```python
from build123d import *

# Parameters (mm, degrees)
SKETCH1_R           = 7.5
BOSS_EXTRUDE1_DEPTH = 58
CUT_EXTRUDE1_REACH  = 42
CUT_EXTRUDE2_REACH  = 82
SKETCH3_R           = 7
CHAMFER1_SIZE       = 15
CUT_EXTRUDE3_DEPTH  = 6
SKETCH4_3_R         = 7.5
CUT_EXTRUDE4_DEPTH  = 12


with BuildPart() as part:
    # Sketch1 → Boss-Extrude1 (new body)
    with BuildSketch(Plane.XY):
        with BuildLine():
            Line((-34, -19), (31, -19))
            Line((31, -19), (46, -10.339745962))
            Line((46, -10.339745962), (46, 12.339745962))
            Line((46, 12.339745962), (31, 21))
            Line((31, 21), (2.66060556, 21))
            ThreePointArc((2.66060556, 21), (-17.33939444, 16.82575695), (-34, 5))
            Line((-34, 5), (-34, -19))
        make_face()
        Circle(SKETCH1_R, mode=Mode.SUBTRACT)
    extrude(amount=BOSS_EXTRUDE1_DEPTH)

    # Sketch2 → Cut-Extrude1 (cut, up to next)
    with BuildSketch(Plane.XZ.offset(19), mode=Mode.PRIVATE) as cut_extrude1_sk1:
        Polygon((-34, 50), (-18, 50), (-18, 44), (20, 44), (20, 14), (-18, 14), (-18, 8), (-34, 8), align=None)
    cut_extrude1_tool1 = extrude(cut_extrude1_sk1.sketch, amount=-CUT_EXTRUDE1_REACH, mode=Mode.PRIVATE) & part.part
    add(cut_extrude1_tool1.solids().sort_by_distance((-9.013245, -19, 29))[0], mode=Mode.SUBTRACT)

    # Sketch3 → Cut-Extrude2 (cut, up to next)
    with BuildSketch(Plane(origin=(46, 0, 0), x_dir=(0, 0, -1), z_dir=(1, 0, 0)), mode=Mode.PRIVATE) as cut_extrude2_sk1:
        with Locations((-29, 1)):
            Circle(SKETCH3_R)
    cut_extrude2_tool1 = extrude(cut_extrude2_sk1.sketch, amount=-CUT_EXTRUDE2_REACH, mode=Mode.PRIVATE) & part.part
    add(cut_extrude2_tool1.solids().sort_by_distance((46, 1, 29))[0], mode=Mode.SUBTRACT)

    # Chamfer1
    chamfer1_edges = [part.edges().sort_by_distance(p)[0] for p in [
        (46, 1, 0),
        (46, 1, 58),
    ]]
    chamfer(chamfer1_edges, length=CHAMFER1_SIZE)

    # Sketch4 → Cut-Extrude3 (cut)
    with BuildSketch(Plane.XY.offset(58)):
        with BuildLine():
            ThreePointArc((-32.533575778, 3.64), (-33.2763294, 2.820381922), (-34, 1.98386677))
            Line((-34, 1.98386677), (-34, -17))
            Line((-34, -17), (-16, -17))
            Line((-16, -17), (-16, 15.224221872))
            ThreePointArc((-16, 15.224221872), (-24.882688852, 10.311155325), (-32.533575778, 3.64))
        make_face()
    extrude(amount=-CUT_EXTRUDE3_DEPTH, mode=Mode.SUBTRACT)

    # Sketch4_3 → Cut-Extrude4 (cut)
    with BuildSketch(Plane.XY.offset(58)):
        with BuildLine():
            Line((-16, 15.224221872), (-16, -17))
            Line((-16, -17), (29, -17))
            Line((29, -17), (29, 19))
            Line((29, 19), (2.66060556, 19))
            ThreePointArc((2.66060556, 19), (-6.858778616, 18.046586751), (-16, 15.224221872))
        make_face()
        Circle(SKETCH4_3_R, mode=Mode.SUBTRACT)
    extrude(amount=-CUT_EXTRUDE4_DEPTH, mode=Mode.SUBTRACT)


solid = part.part
```
Read the model definition and answer for the solid it produces. Units are mm, in the model's axes. A direction names the side the tool comes from. Coordinates: 2 decimals unless noted, no trailing zeros. Order: outer loops, then holes, each group sorted by start corner. A loop starts at its lowest first (then second) coordinate and runs counter-clockwise, first axis right, second up. Notation, with made-up numbers: (-16.75, -22.5) - (30.25, -22.5) arc R17 ccw to (30.25, -5.5) - close; hole circle Ø11 at (73.25, 87.25). An arc over 180 degrees is marked (long way). Answer as a JSON object with one key per item and string values. Group by question number.
Item 1: The mould has two halves that part along X. Classify faces 4 (the face through (-25, -4, 52)), 5 (the face through (36.73, -15.69, 28.59)), 6 (the face through (33.182, 3.103, 22.323)), 7 (the face through (4, -17, 52)): +X half, -X half, draft (parallel to the pull), parting line (faces both ways), or undercut.
Item 2: Section D-D (y = 0) is taken. State how many separate pieces and enclosed holes the cut face has, plus the area to 3 significant figures.
Item 3: Consider probe 1 along Z at (x, y) = (12, 4); probe 2 along Z at (x, y) = (-27, -3); probe 3 along Y at (x, z) = (21, 55). Determine where each line is inside the solid, lowest interval first. Write a range as from..to.
Item 4: Section A-A (z = 29) is taken. Give the vertices of the cut face in (x, y).
Item 5: Section C-C (x = 28) is taken. Give the vertices of the cut face in (y, z), plus the area to 3 significant figures.
Item 6: Section B-B (x = -22) is taken. Give the vertices of the cut face in (y, z), plus the area to 3 significant figures.
Item 7: Flat-ended cylindrical pins translate along their axes: P1, Ø3, axis at y = -2, z = 10, coming from the -X side; P2, Ø15, axis at y = 10, z = 31, coming from the -X side; P3, Ø12.5, axis at y = 1, z = 29, coming from the -X side; P4, Ø12, axis at x = 10.5, y = -9.5, coming from the -Z side. Find the tip coordinate at first contact, or state that the pin passes through.
Item 8: A tool of negligible diameter and unlimited length cuts with its end or side. For faces 1 (the face through (-26, -5, 8)), 2 (the face through (11, 1, 46)), 3 (the face through (-34, -7, 51)), from which of +Z, -Z, +X, -X, +Y, -Y can it reach the whole face along a straight path? Write none if from no direction.
Results are:
{
 "1": {"face 4": "undercut", "face 5": "+X half", "face 6": "draft", "face 7": "undercut"},
 "2": {"separate pieces": "4", "enclosed holes": "0", "area": "1,350 mm^2"},
 "3": {"probe 1": "z = 0..14, 44..46", "probe 2": "z = 0..8, 50..52", "probe 3": "y = -19..-17, 19..21"},
 "4": {"outline": "(20, -19) - (31, -19) - (46, -10.34) - (46, -6) - (20, -6) - close; (20, 8) - (46, 8) - (46, 12.34) - (31, 21) - (20, 21) - close"},
 "5": {"outline": "(-19, 0) - (21, 0) - (21, 58) - (19, 58) - (19, 46) - (-17, 46) - (-17, 58) - (-19, 58) - close; hole circle Ø14 at (1, 29)", "area": "1,730 mm^2"},
 "6": {"outline": "(-19, 0) - (14.5, 0) - (14.5, 8) - (-19, 8) - close; (-19, 50) - (14.5, 50) - (14.5, 58) - (12.18, 58) - (12.18, 52) - (-17, 52) - (-17, 58) - (-19, 58) - close", "area": "361 mm^2"},
 "7": {"P1": "stops at x = -18", "P2": "stops at x = 20", "P3": "passes through", "P4": "stops at z = 0"},
 "8": {"face 1": "-X, +Y, -Y", "face 2": "+Z", "face 3": "+Z, -Z, -X, +Y, -Y"}
}
